from build123d import *

# Parameters (mm, degrees)
SKETCH_1_W      = 12
SKETCH_1_H      = 12
EXTRUDE_1_DEPTH = 3
SKETCH_2_W      = 5
SKETCH_2_H      = 5
EXTRUDE_2_DEPTH = 3.4
SKETCH_3_R      = 6.5
EXTRUDE_3_DEPTH = 1
EXTRUDE_START   = -7.4
SKETCH_4_R      = 5.85
EXTRUDE_4_DEPTH = 12
SKETCH_5_W      = 0.2
SKETCH_5_H      = 0.9
EXTRUDE_5_DEPTH = 5


with BuildPart() as part:
    # 草图1 → 凸台-拉伸1 (new body)
    with BuildSketch(Plane(origin=(0, 0, 0), x_dir=(1, 0, 0), z_dir=(0, 1, 0))):
        Rectangle(SKETCH_1_W, SKETCH_1_H)
    extrude(amount=EXTRUDE_1_DEPTH)

    # 草图2 → 凸台-拉伸2 (add)
    with BuildSketch(Plane(origin=(0, 3, 0), x_dir=(1, 0, 0), z_dir=(0, 1, 0))):
        Rectangle(SKETCH_2_W, SKETCH_2_H)
    extrude(amount=EXTRUDE_2_DEPTH)

    # 草图3 → 凸台-拉伸3 (add)
    with BuildSketch(Plane(origin=(0, 6.4, 0), x_dir=(1, 0, 0), z_dir=(0, 1, 0))):
        Circle(SKETCH_3_R)
    extrude(amount=EXTRUDE_3_DEPTH)

    # 草图4 → 凸台-拉伸4 (add)
    with BuildSketch(Plane(origin=(0, 7.4, 0), x_dir=(1, 0, 0), z_dir=(0, 1, 0)).offset(EXTRUDE_START)):
        Circle(SKETCH_4_R)
    extrude(amount=EXTRUDE_4_DEPTH)

    # 草图5 → 凸台-拉伸5 (add)
    with BuildSketch(Plane.XZ):
        with Locations((5.9, 2.55)):
            Rectangle(SKETCH_5_W, SKETCH_5_H)
        with Locations((5.9, -2.55)):
            Rectangle(SKETCH_5_W, SKETCH_5_H)
        with Locations((-5.9, -2.55)):
            Rectangle(SKETCH_5_W, SKETCH_5_H)
        with Locations((-5.9, 2.55)):
            Rectangle(SKETCH_5_W, SKETCH_5_H)
    extrude(amount=EXTRUDE_5_DEPTH)


solid = part.part
Can you work these out from the model? Positions are in its coordinate system, mm. A direction names the side the tool comes from. Coordinates: 2 decimals unless noted, no trailing zeros. Loops run counter-clockwise (first coordinate to the right, second up) from the corner with the lowest first, then second, coordinate; pieces in that order, holes last. Notation, with made-up numbers: M 7.25,-19.5 L 13.25,-19.5 A25 ccw 13.25,2.5 Z; hole C 28,-28 d11. An arc over 180 degrees is marked long. Answer as CSV lines item,"result". Start each with the question number.
1. If I drill on probe 1 along X at (y, z) = (0.5, -4.25); probe 2 along Y at (x, z) = (-5, -2), over which ranges is the centre line in solid material (lowest first)? Write a range as [from, to].
2. For pin 1 Ø1 at (y, z) = (10, 1.5) entering from -X; pin 2 Ø1.5 at (x, y) = (-0.5, 1) entering from -Z; pin 3 Ø4 at (x, z) = (-2.5, 3) entering from -Y, each with a flat end and sliding along its axis, tell me the tip position at first contact or that it passes through.
3. Suppose I cut it at D-D, the plane y = 3.5. List the corners of the cut face in (x, z) for me.
4. Suppose I cut it at C-C, the plane x = 0. List the corners of the cut face in (y, z) for me.
5. Thinking about a two-plate mould opening in Y: for faces 4 (the face through (0, 12, 0)), 5 (the face through (5.8, -2.5, -2.6)), 6 (the face through (-1.81, 3, 5.75)), which applies, +Y half, -Y half, draft (parallel to the pull), parting line (faces both ways), or undercut?
6. Suppose I cut it at A-A, the plane y = -3. List the corners of the cut face in (x, z) for me, plus the area to 3 significant figures.
7. For faces 1 (the face through (-5.8, -2.5, 2.5)), 2 (the face through (-6, 1, 0)), 3 (the face through (6, 1, 0)), which set-ups out of +Z, -Z, +X, -X, +Y, -Y let a thin tool reach every point of the face, with its end or its side?
8. Suppose I cut it at B-B, the plane z = 0. List the corners of the cut face in (x, y) for me, plus the area to 3 significant figures.
Output:
1,probe 1,"x = [-6, 6]"
1,probe 2,"y = [0, 12]"
2,pin 1,"stops at x = -5.76"
2,pin 2,"stops at z = -6"
2,pin 3,"stops at y = 0"
3,outline,"C 0,0 d11.7"
4,outline,"M 0,-6 L 3,-6 L 3,-5.85 L 6.4,-5.85 L 6.4,-6.5 L 7.4,-6.5 L 7.4,-5.85 L 12,-5.85 L 12,5.85 L 7.4,5.85 L 7.4,6.5 L 6.4,6.5 L 6.4,5.85 L 3,5.85 L 3,6 L 0,6 Z"
5,face 4,"+Y half"
5,face 5,"draft"
5,face 6,"undercut"
6,outline,"M -6,-3 L -5.8,-3 L -5.8,-2.1 L -6,-2.1 Z; M -6,2.1 L -5.8,2.1 L -5.8,3 L -6,3 Z; M 5.8,-3 L 6,-3 L 6,-2.1 L 5.8,-2.1 Z; M 5.8,2.1 L 6,2.1 L 6,3 L 5.8,3 Z"
6,area,"0.720 mm^2"
7,face 1,"+Z, -Z, -Y"
7,face 2,"+Z, -Z, -X, -Y"
7,face 3,"+Z, -Z, +X, -Y"
8,outline,"M -6.5,6.4 L -5.85,6.4 L -5.85,3 L -6,3 L -6,0 L 6,0 L 6,3 L 5.85,3 L 5.85,6.4 L 6.5,6.4 L 6.5,7.4 L 5.85,7.4 L 5.85,12 L -5.85,12 L -5.85,7.4 L -6.5,7.4 Z"
8,area,"143 mm^2"
